Design review of the part built by this model. Coordinates are the model's own, in mm. A direction names the side the tool comes from. Give positions to 0.01 mm unless a question says otherwise; leave off trailing zeros. Write each loop counter-clockwise with the first axis right and the second up, starting at its lowest first coordinate (ties: lowest second). Pieces come first, ordered by that corner, then holes. Notation, with made-up numbers: (-9.5, -10) -> (16.5, -10) arc R6 cw to (16.5, -5) -> close; hole circle Ø11 at (64.5, 13.5). An arc over 180 degrees is marked (long way). Put each result on its own line as item: value. Start each with the question number.
from build123d import *

# Parameters (mm, degrees)
F0_R     = 6.35
F1_DEPTH = 25.4
F2_R     = 12.7
F2_R_2   = 6.35
F3_DEPTH = 203.2
F4_R     = 6.35
F5_DEPTH = 25.4


with BuildPart() as f1:
    # F0 (on Front) → F1 (new body)
    with BuildSketch(Plane.XZ):
        Circle(F0_R)
    extrude(amount=F1_DEPTH)

    # F2 (on face) → F3 (join)
    with BuildSketch(Plane.XZ.offset(25.4)):
        Circle(F2_R)
        Circle(F2_R_2, mode=Mode.SUBTRACT)
        Circle(F2_R_2)
    extrude(amount=F3_DEPTH)

    # F4 (on face) → F5 (join)
    with BuildSketch(Plane.XZ.offset(228.6)):
        Circle(F4_R)
    extrude(amount=F5_DEPTH)


solid = f1.part
Q1. For pin 1 (4 mm diameter, centred on x = 7, y = -200.5, fed in from +Z); pin 2 (5 mm diameter, centred on y = -88, z = -4, fed in from -X); pin 3 (3 mm diameter, centred on x = -4.5, y = -111.5, fed in from +Z), all flat-tipped, find the tip position at first contact; note any pin that passes through.
Q2. Machinability: for faces 3 (the face through (-1.38, -12.52, -6.2)), 4 (the face through (0, 0, 0)), 5 (the face through (3, -228.6, 6)), which of the approach directions +Z, -Z, +X, -X, +Y, -Y give a long, thin tool a straight path to every point of the face, cutting with its end or side? Answer none if there is none.
Q3. Take a section at B-B on z = 0. Give the boundary of the cut face in (x, y).
Q4. Take a section at C-C on y = -72.5. Give the boundary of the cut face in (x, z).
Q5. Mouldability with a two-part tool opening along Z and no side actions: class faces 1 (the face through (-2.75, -125.58, -12.4)), 2 (the face through (3, -25.4, 6)) as +Z half, -Z half, draft (parallel to the pull), parting line (faces both ways), or undercut.
Q6. To check wall thickness, follow probe 1 along Y at (x, z) = (-4, -6.5); probe 2 along Z at (x, y) = (-0.5, -22.5); probe 3 along X at (y, z) = (-139, -2.75). State the ranges of each line that lie inside material, in increasing order. Write a range as from..to.
Q7. Take a section at A-A on x = 0. Give the boundary of the cut face in (y, z).
Result:
1. pin 1: stops at z = 11.67
1. pin 2: stops at x = -12.61
1. pin 3: stops at z = 12.34
2. face 3: +Y
2. face 4: +Z, -Z, +X, -X, +Y
2. face 5: -Y
3. outline: (-12.7, -228.6) -> (-6.35, -228.6) -> (-6.35, -254) -> (6.35, -254) -> (6.35, -228.6) -> (12.7, -228.6) -> (12.7, -25.4) -> (6.35, -25.4) -> (6.35, 0) -> (-6.35, 0) -> (-6.35, -25.4) -> (-12.7, -25.4) -> close
4. outline: circle Ø25.4 at (0, 0)
5. face 1: parting line
5. face 2: draft
6. probe 1: y = -228.6..-25.4
6. probe 2: z = -6.33..6.33
6. probe 3: x = -12.4..12.4
7. outline: (-254, -6.35) -> (-228.6, -6.35) -> (-228.6, -12.7) -> (-25.4, -12.7) -> (-25.4, -6.35) -> (0, -6.35) -> (0, 6.35) -> (-25.4, 6.35) -> (-25.4, 12.7) -> (-228.6, 12.7) -> (-228.6, 6.35) -> (-254, 6.35) -> close
